Autodesk Inventor part; units mm, degrees
ref_plane "Work Plane1" through (0, 0, -15) normal (0, 0, 1) x (1, 0, 0)
ref_plane "YZ Plane" through (0, 0, 0) normal (1, 0, 0) x (0, 1, 0)
ref_plane "XZ Plane" through (0, 0, 0) normal (0, 1, 0) x (-1, 0, 0)
sketch "Sketch1" plane through (0, 0, 0) normal (0, 0, 1) x (1, 0, 0)
  line L0 (0, 0) -> (25, 0)
  line L1 (25, 0) -> (25, 40)
  line L2 (25, 40) -> (0, 40)
  line L3 (0, 40) -> (0, 0)
  dimension "d1" = 25
  dimension "d2" = 40
  dimension "d3" = 25
extrude "Extrusion1" add sketch "Sketch1" against normal blind 30
sketch "Sketch2" plane through (25, 0, 0) normal (1, 0, 0) x (0, 0, -1)
  line L0 (0, 0) -> (30, 0)
  circle A0 centre (15, 6.56) radius 2.46
extrude "Extrusion2" cut sketch "Sketch2" against normal blind 30
sketch "Sketch3" plane through (0, 0, 0) normal (-1, 0, 0) x (0, 0, 1)
  line L0 (0, 0) -> (-30, 0)
  line L1 (-25.05, 0) -> (-4.95, 0)
  line L2 (-4.95, 0) -> (-4.95, 33.12)
  line L3 (-4.95, 33.12) -> (-25.05, 33.12)
  line L4 (-25.05, 33.12) -> (-25.05, 0)
  dimension "d11" = 20.1
extrude "Extrusion3" cut sketch "Sketch3" against normal blind 20
sketch "Sketch4" plane through (0, 0, 0) normal (0, -1, 0) x (1, 0, 0)
  line L0 (20, -4.95) -> (20, -25.05)
  line L1 (20, -15) -> (25, -15)
  line L2 (25, 0) -> (25, -30)
  line L3 (20, -8.025) -> (25, -8.025)
  line L4 (25, -8.025) -> (25, -21.975)
  line L5 (25, -21.975) -> (20, -21.975)
  line L6 (20, -21.975) -> (20, -8.025)
  line L7 (20, -8.025) -> (25, -21.975) construction
  line L8 (25, -8.025) -> (20, -21.975) construction
  line L9 (25, -12.54) -> (25, -17.46)
  point P0 (0, 0)
  point P1 (22.5, -15)
  dimension "d14" = 13.95
extrude "Extrusion4" add sketch "Sketch4" along normal blind 15
sketch "Sketch5" plane through (20, 0, 0) normal (-1, 0, 0) x (0, 0, 1)
  circle A0 centre (-15, 6.56) radius 2.46
  circle A1 centre (-15, 6.56) radius 4.7025
  circle A2 centre (-15, 6.56) radius 2.46
  circle A3 centre (-15, 6.56) radius 2.46
  point P0 (0, 0)
  dimension "d17" = 9.405
extrude "Extrusion5" cut sketch "Sketch5" against normal blind 2.1
sketch "Sketch6" plane through (25, 0, 0) normal (1, 0, 0) x (0, 0, -1)
  circle A0 centre (15, 6.56) radius 4.7025
  line L0 (15, 6.56) -> (15, 23.56)
  circle A1 centre (15, 23.56) radius 2.46
  point P0 (0, 0)
  dimension "d20" = 17
  dimension "d21" = 4.92
extrude "Extrusion6" cut sketch "Sketch6" against normal blind 10 contours A1
sketch "Sketch7" plane through (20, 0, 0) normal (-1, 0, 0) x (0, 0, 1)
  circle A0 centre (-15, 23.56) radius 2.46
  circle A1 centre (-15, 23.56) radius 4.7025
  point P0 (0, 0)
  dimension "d24" = 9.405
extrude "Extrusion7" cut sketch "Sketch7" against normal blind 2.1
sketch "Sketch9" plane through (25, 0, 0) normal (1, 0, 0) x (0, 0, -1)
  circle A0 centre (15, 6.56) radius 2.46
  circle A1 centre (15, 6.56) radius 2.46
  circle A2 centre (15, 23.56) radius 2.46
  circle A3 centre (15, 23.56) radius 2.46
  line L0 (30, 40) -> (30, 0)
  line L1 (30, 0) -> (30, 40)
  line L2 (30, 40) -> (0, 40)
  line L3 (0, 40) -> (0, 0)
  line L4 (0, 0) -> (8.025, 0)
  line L5 (21.975, 0) -> (21.975, -15)
  line L6 (21.975, -15) -> (8.025, -15)
  line L7 (8.025, -15) -> (8.025, 0)
  line L8 (0, 0) -> (8.025, 0)
  line L9 (21.975, 0) -> (30, 0)
extrude "Extrusion8" add sketch "Sketch9" along normal blind 5
sketch "Sketch10" plane through (0, 40, 0) normal (0, 1, 0) x (1, 0, 0)
  line L0 (0, 30) -> (30, 30)
  line L1 (30, 0) -> (0, 0)
  line L2 (0, 30) -> (30, 30)
  line L3 (30, 30) -> (30, 0)
  line L4 (30, 0) -> (0, 0)
  line L5 (0, 0) -> (0, 30)
extrude "Extrusion9" add sketch "Sketch10" along normal blind 30
sketch "Sketch12" plane through (30, 0, 0) normal (1, 0, 0) x (0, 0, -1)
  circle A0 centre (15, 6.56) radius 2.46
  line L0 (15, 6.56) -> (15, 15.06)
  circle A1 centre (15, 15.06) radius 2.525
  point P0 (0, 0)
  dimension "d31" = 8.5
  dimension "d33" = 5.05
extrude "Extrusion10" cut sketch "Sketch12" against normal blind 30 contours A1
sketch "Sketch15" plane through (0, 0, -25.05) normal (-1, 0, 0) x (0, 0, 1)
  line L0 (0, 33.12) -> (20.1, 33.12)
  line L1 (20.1, 33.12) -> (20.1, 0)
  line L2 (0, 33.12) -> (20.1, 33.12)
  line L3 (20.1, 33.12) -> (20.1, 31.1)
  line L4 (20.1, 31.1) -> (0, 31.1)
  line L5 (0, 31.1) -> (0, 33.12)
  point P0 (25.05, 0)
  dimension "d57" = 2.02
extrude "Extrusion13" add sketch "Sketch15" against normal blind 20
sketch "Sketch17" plane through (0, 0, 0) normal (0, 0, 1) x (1, 0, 0)
  line L0 (0, 70) -> (30, 70)
  line L1 (30, 70) -> (50.0622, 90.0622)
  line L2 (30, 70) -> (80, 70) construction
  line L3 (11.9522, 97.2454) -> (0, 85.2932)
  line L4 (0, 70) -> (0, 85.2932)
  line L5 (0, 70) -> (0, 0)
  line L6 (0, 70) -> (30, 70)
  line L7 (10.923, 112.2849) -> (0, 120.567)
  line L8 (50.0622, 105.3553) -> (50.0622, 120.567)
  line L9 (50.0622, 105.3553) -> (50.0622, 90.0622)
  arc A0 (11.9522, 97.2454) -> (10.923, 112.2849) centre (4.8811, 104.3165) ccw
  line L10 (0, 156.567) -> (30, 156.567)
  line L11 (30, 156.567) -> (50.0622, 120.567)
  line L12 (5, 154.567) -> (0, 156.567)
  line L13 (5, 122.567) -> (0, 120.567)
  line L14 (5, 122.567) -> (10, 138.567)
  line L15 (10, 138.567) -> (5, 154.567)
  dimension "d61" = 45
  dimension "d62" = 32.0271
  dimension "d72" = 10
extrude "Extrusion14" add sketch "Sketch17" against normal blind 30
sketch "Sketch23" plane through (0, 0, 0) normal (0, 0, 1) x (1, 0, 0)
  line L0 (50.0622, 90.0622) -> (30, 70)
  line L1 (30, 70) -> (50.0622, 90.0622)
  line L2 (50.0622, 120.567) -> (50.0622, 90.0622)
  line L3 (50.0622, 90.0622) -> (50.0622, 120.567)
  line L4 (30, 156.567) -> (50.0622, 120.567)
  line L5 (50.0622, 120.567) -> (30, 156.567)
  line L6 (0, 156.567) -> (30, 156.567)
  line L7 (30, 156.567) -> (0, 156.567)
  line L8 (5, 154.567) -> (0, 156.567)
  line L9 (0, 156.567) -> (5, 154.567)
  line L10 (10, 138.567) -> (5, 154.567)
  line L11 (5, 154.567) -> (10, 138.567)
  line L12 (5, 122.567) -> (10, 138.567)
  line L13 (10, 138.567) -> (5, 122.567)
  line L14 (0, 120.567) -> (5, 122.567)
  line L15 (5, 122.567) -> (0, 120.567)
  line L16 (10.923, 112.2849) -> (0, 120.567)
  line L17 (0, 120.567) -> (10.923, 112.2849)
  line L18 (0, 85.2932) -> (11.9522, 97.2454)
  line L19 (11.9522, 97.2454) -> (0, 85.2932)
  line L20 (0, 85.2932) -> (0, 55.2932)
  line L21 (0, 0) -> (0, 85.2932)
  line L22 (0, 55.2932) -> (30, 55.2932)
  line L23 (30, 0) -> (30, 70)
  line L24 (30, 55.2932) -> (30, 70)
  arc A0 (11.9522, 97.2454) -> (10.923, 112.2849) centre (4.8811, 104.3165) ccw
  dimension "d97" = 30
extrude "Extrusion15" add sketch "Sketch23" along normal blind 15
ref_plane "Work Plane1" through (0, 0, -15) normal (0, 0, 1) x (1, 0, 0)
mirror "Mirror1" about plane through (0, 0, -15) normal (0, 0, 1) of "Extrusion15"
properties part number "rec_c_32mm_x_60mm"
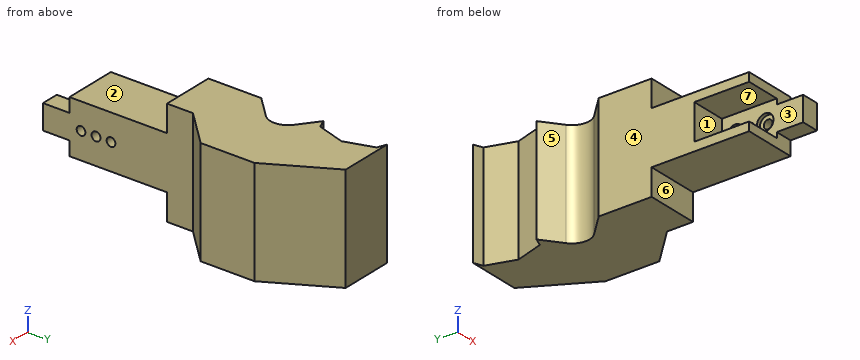
Model file for the job. Use its own axes, mm. Face numbers are marked on the shaded views. A direction names the side the tool comes from. Coordinates: 2 decimals unless noted, no trailing zeros. Loops run counter-clockwise (first coordinate to the right, second up) from the corner with the lowest first, then second, coordinate; pieces in that order, holes last. Notation, with made-up numbers: (-3, 9.25) - (4, 9.25) arc R27 cw to (4, 36.25) - close; hole circle Ø1 at (39, 28). An arc over 180 degrees is marked (long way). Answer as a JSON object with one key per item and string values. Group by question number.
(1) Cut at D-D (y = 60.5). Give the cut face in (x, z), then the cut area to 3 significant figures.
(2) Probe line 1 along Y through (x, z) = (28.5, -15) (3 decimals); line 2 along Y through (x, z) = (20.7, -15) (1 decimal); line 3 along Z through (x, y) = (21, 6). List the from-to ranges inside material, lowest first.
(3) Cut at C-C (x = 8). Give the cut face in (y, z).
(4) Cut at B-B (x = 26.5). Give the cut face in (y, z) (3 decimals).
(5) Flat gauge pins, fed straight in: pin 1 (12 mm diameter, centred on y = 6.56, z = -15, fed in from -X); pin 2 (3 mm diameter, centred on y = 23.56, z = -15, fed in from -X); pin 3 (3 mm diameter, centred on y = 46.5, z = -25, fed in from +X); pin 4 (4.5 mm diameter, centred on y = 4.5, z = -15.5, fed in from -X). Where does each tip first touch, or does it go through?
(6) Two-plate mould, pull along Z, no slides. Class the marked faces 1, 2, 3 and 4: released by +Z, released by -Z, zero draft, split by the parting line, or undercut.
(7) Cut at A-A (y = 15.06). Give the cut face in (x, z) (3 decimals).
(8) Tool access for the marked faces 5, 6 and 7: list every direction of +Z, -Z, +X, -X, +Y, -Y with a clear straight run to the whole face (end or side of a thin tool).
Geometry says:
{
 "1": {"outline": "(0, -45) - (30, -45) - (30, 15) - (0, 15) - close", "area": "1,800 mm^2"},
 "2": {"line 1": "y = -15 to 4.1, 9.02 to 12.535, 17.585 to 21.1, 26.02 to 156.567", "line 2": "y = -15 to 1.9, 11.3 to 12.5, 17.6 to 18.9, 28.3 to 156.6", "line 3": "z = -30 to -19.67, -10.33 to 0"},
 "3": {"outline": "(0, -30) - (55.29, -30) - (55.29, -45) - (93.29, -45) - (93.29, 15) - (55.29, 15) - (55.29, 0) - (0, 0) - (0, -4.95) - (31.1, -4.95) - (31.1, -25.05) - (0, -25.05) - close; (114.5, -45) - (132.17, -45) - (132.17, 15) - (114.5, 15) - close; (144.97, -45) - (156.57, -45) - (156.57, 15) - (144.97, 15) - close"},
 "4": {"outline": "(-15, -21.975) - (0, -21.975) - (0, -30) - (55.293, -30) - (55.293, -45) - (156.567, -45) - (156.567, 15) - (55.293, 15) - (55.293, 0) - (0, 0) - (0, -8.025) - (-15, -8.025) - close; hole circle Ø4.92 at (6.56, -15); hole circle Ø5.05 at (15.06, -15); hole circle Ø4.92 at (23.56, -15)"},
 "5": {"pin 1": "stops at x = 20", "pin 2": "passes through", "pin 3": "stops at x = 30", "pin 4": "stops at x = 22.1"},
 "6": {"face 1": "undercut", "face 2": "released by +Z", "face 3": "undercut", "face 4": "zero draft"},
 "7": {"outline": "(0, -30) - (30, -30) - (30, -17.525) - (20, -17.525) - (20, -25.05) - (0, -25.05) - close; (0, -4.95) - (20, -4.95) - (20, -12.475) - (30, -12.475) - (30, 0) - (0, 0) - close"},
 "8": {"face 5": "+Z, -Z, -X", "face 6": "-Z, +X, -X, -Y", "face 7": "-X, -Y"}
}
